Verification items for this drawing (mm, ordinates from the low corner). Round coordinates to 2 decimals unless told otherwise and drop trailing zeros. Loops run counter-clockwise (first coordinate to the right, second up) from the corner with the lowest first, then second, coordinate; pieces in that order, holes last. Notation, with made-up numbers: (68, -28.5) -> (111, -28.5) arc R14 cw to (111, -16.5) -> close; hole circle Ø11 at (46.25, -31). An arc over 180 degrees is marked (long way). One line per item, written item: value. Start each with the question number.
1. Material ranges on L1, parallel to X at y = 17.5, z = 1.95, recorded low to high.
2. Cross-section at A-A on z = 1.8. Record the cut outline in (x, y), then the cut area to 3 significant figures.
3. Cross-section at B-B on y = 19. Record the cut outline in (x, z), then the cut area to 3 significant figures.
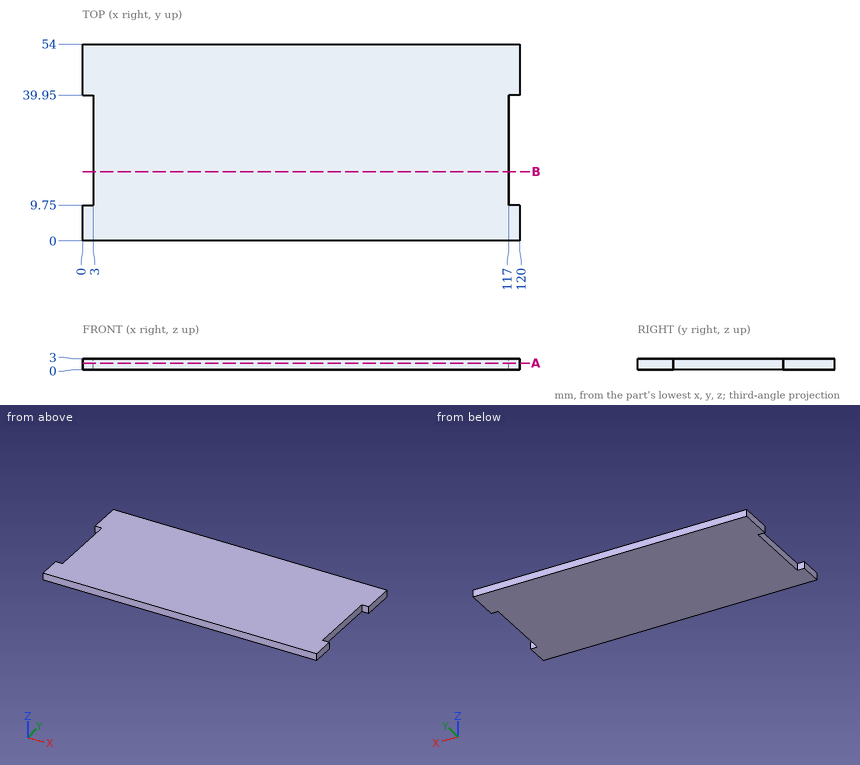
Taken from the geometry:
1. L1: x = 3 to 117
2. outline: (0, 0) -> (120, 0) -> (120, 9.75) -> (117, 9.75) -> (117, 39.95) -> (120, 39.95) -> (120, 54) -> (0, 54) -> (0, 39.95) -> (3, 39.95) -> (3, 9.75) -> (0, 9.75) -> close
2. area: 6,300 mm2
3. outline: (3, 0) -> (117, 0) -> (117, 3) -> (3, 3) -> close
3. area: 342 mm2
